The model under review builds one solid part; all positions refer to its coordinate system, in mm. Round coordinates to 2 decimals unless told otherwise and drop trailing zeros. Loops run counter-clockwise (first coordinate to the right, second up) from the corner with the lowest first, then second, coordinate; pieces in that order, holes last. Notation, with made-up numbers: (-39, 4) -> (16, 4) arc R24 cw to (16, 33) -> close; hole circle Ø2 at (7.5, 47). An arc over 180 degrees is marked (long way). Use CSV: the item, a comma, the result in double quotes. Start each with the question number.
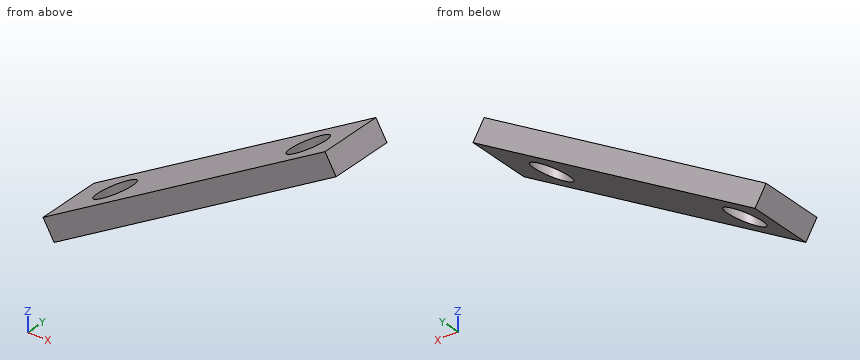
```python
from build123d import *

# Parameters (mm, degrees)
F2_DEPTH = 15
F0_R     = 8
F3_DEPTH = 81.984738


with BuildPart() as f2:
    # F1 (on Front) → F2 (new body, symmetric)
    with BuildSketch(Plane.XZ):
        Polygon((122, 81.983738), (-5, 8.660254), (0, 0), (127, 73.323484), align=None)
    extrude(amount=F2_DEPTH, both=True)

    # F0 (on Top) → F3 (cut, through all)
    with BuildSketch(Plane.XY):
        with Locations((16, 0)):
            Circle(F0_R)
        with Locations((103, 0)):
            Circle(F0_R)
    extrude(amount=F3_DEPTH, mode=Mode.SUBTRACT)


solid = f2.part
```
1. Take a section at B-B, the plane y = 3. Give the boundary of the cut face in (x, z).
2. Take a section at D-D, the plane z = 11. Give the boundary of the cut face in (x, y), then the cut area to 3 significant figures.
3. For line 1 along Y through (x, z) = (16, 10.75); line 2 along Z through (x, y) = (92, 0.75); line 3 along Z through (x, y) = (2.5, -6.5), list the stretches that pass through material, from the lowest coordinate up. Write a range as from..to.
4. Clearance check with flat-ended pins moving along their axes: P1, Ø6, axis at x = 26.5, y = 1, coming from the +Z side; P2, Ø8, axis at y = 3, z = 27, coming from the +X side; P3, Ø10, axis at y = -1, z = 10.5, coming from the -X side; P4, Ø5, axis at x = 86, z = 64, coming from the +Y side. State where each tip first meets the part, or that it passes through.
5. Take a section at A-A, the plane x = 103. Give the boundary of the cut face in (y, z), then the cut area to 3 significant figures.
6. Take a section at C-C, the plane y = 9.75. Give the boundary of the cut face in (x, z), then the cut area to 3 significant figures.
Results:
1,outline,"(-5, 8.66) -> (0, 0) -> (8.58, 4.96) -> (8.58, 16.5) -> close; (23.42, 13.52) -> (95.58, 55.19) -> (95.58, 66.73) -> (23.42, 25.07) -> close; (110.42, 63.75) -> (127, 73.32) -> (122, 81.98) -> (110.42, 75.3) -> close"
2,outline,"(-0.95, -15) -> (19.05, -15) -> (19.05, -7.39) arc R8 cw (long way) to (19.05, 7.39) -> (19.05, 15) -> (-0.95, 15) -> close"
2,area,"452 mm²"
3,line 1,"-15..-8, 8..15"
3,line 2,"53.12..64.66"
3,line 3,"1.44..12.99"
4,P1,"z = 28.58"
4,P2,"x = 53.69"
4,P3,"x = -5"
4,P4,"y = 15"
5,outline,"(-15, 59.47) -> (-8, 59.47) -> (-8, 71.01) -> (-15, 71.01) -> close; (8, 59.47) -> (15, 59.47) -> (15, 71.01) -> (8, 71.01) -> close"
5,area,"162 mm²"
6,outline,"(-5, 8.66) -> (0, 0) -> (127, 73.32) -> (122, 81.98) -> close"
6,area,"1,470 mm²"
